The listing builds one solid part. Answer for the finished solid, in the listing's coordinates (mm). Coordinates: 2 decimals unless noted, no trailing zeros. Order: outer loops, then holes, each group sorted by start corner. A loop starts at its lowest first (then second) coordinate and runs counter-clockwise, first axis right, second up. Notation, with made-up numbers: (77.25, 14) -> (93.25, 14) arc R14 cw to (93.25, 28) -> close; hole circle Ø5 at (47.5, 33). An arc over 180 degrees is marked (long way). One line per question, with ' | ' between items.
from build123d import *

# Parameters (mm, degrees)
BOSS_EXTRUDE1_DEPTH    = 25.4
CUT_EXTRUDE1_DEPTH     = 25.4
F_1_1_DIAMETER_HOLE1_D = 25.4


with BuildPart() as part:
    # Sketch1 → Boss-Extrude1 (new body)
    with BuildSketch(Plane.XY):
        with BuildLine():
            Line((-196.85, -171.45), (196.85, -171.45))
            ThreePointArc((196.85, -171.45), (220.423172318, -161.685672318), (230.1875, -138.1125))
            Line((230.1875, -138.1125), (230.1875, 138.1125))
            ThreePointArc((230.1875, 138.1125), (220.423172318, 161.685672318), (196.85, 171.45))
            Line((196.85, 171.45), (-196.85, 171.45))
            ThreePointArc((-196.85, 171.45), (-220.423172318, 161.685672318), (-230.1875, 138.1125))
            Line((-230.1875, 138.1125), (-230.1875, -138.1125))
            ThreePointArc((-230.1875, -138.1125), (-220.423172318, -161.685672318), (-196.85, -171.45))
        make_face()
    extrude(amount=BOSS_EXTRUDE1_DEPTH)

    # Sketch2 → Cut-Extrude1 (cut)
    with BuildSketch(Plane.XY.offset(25.4)):
        with BuildLine():
            Line((-230.1875, 138.1125), (-230.1875, -138.1125))
            ThreePointArc((-230.1875, -138.1125), (-220.423172318, -161.685672318), (-196.85, -171.45))
            Line((-196.85, -171.45), (-122.025168103, -171.45))
            ThreePointArc((-122.025168103, -171.45), (-145.59834042, -161.685672318), (-155.362668103, -138.1125))
            Line((-155.362668103, -138.1125), (-155.362668103, 139.975839194))
            ThreePointArc((-155.362668103, 139.975839194), (-145.020467472, 162.332230308), (-122.137381725, 171.45))
            Line((-122.137381725, 171.45), (-155.460095347, 171.45))
            Line((-155.460095347, 171.45), (-196.85, 171.45))
            ThreePointArc((-196.85, 171.45), (-220.423172318, 161.685672318), (-230.1875, 138.1125))
        make_face()
    extrude(amount=-CUT_EXTRUDE1_DEPTH, mode=Mode.SUBTRACT)

    # 1 (1) Diameter Hole1 (through all)
    with Locations(Plane.XY.offset(25.4)):
        with Locations((25.4, 0), (-36.924961559, 107.95), (87.724961559, 107.95), (150.049923118, 0), (87.724961559, -107.95), (-36.924961559, -107.95), (-99.249923118, 0)):
            Hole(F_1_1_DIAMETER_HOLE1_D / 2)


solid = part.part
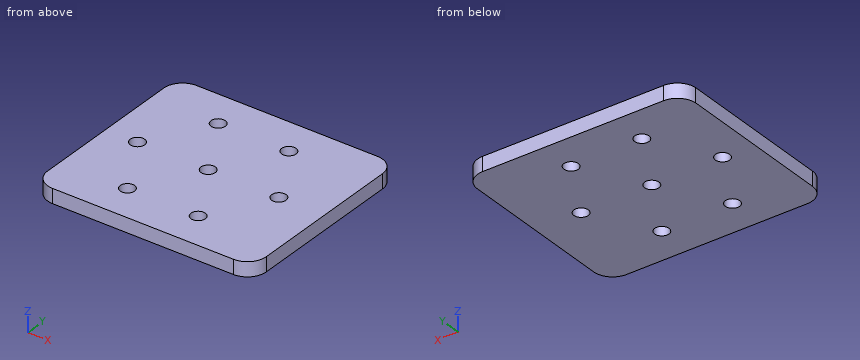
Item 1: Section A-A, the plane x = 25.4 is taken. Give the vertices of the cut face in (y, z).
Computed values:
outline: (-171.45, 0) -> (-12.7, 0) -> (-12.7, 25.4) -> (-171.45, 25.4) -> close; (12.7, 0) -> (171.45, 0) -> (171.45, 25.4) -> (12.7, 25.4) -> close
Item 2: This flat-tipped pin is pushed along its axis until it touches: pin 1 Ø20.5 at (x, y) = (-36.92, 107.95) entering from +Z. Where does it stop, or does it pass through?
Computed values:
pin 1: passes through
Item 3: Section B-B, the plane y = -107.95 is taken. Give the vertices of the cut face in (x, z), plus the area to 3 significant figures.
Computed values:
outline: (-155.36, 0) -> (-49.62, 0) -> (-49.62, 25.4) -> (-155.36, 25.4) -> close; (-24.22, 0) -> (75.02, 0) -> (75.02, 25.4) -> (-24.22, 25.4) -> close; (100.42, 0) -> (230.19, 0) -> (230.19, 25.4) -> (100.42, 25.4) -> close | area: 8,500 mm^2
Item 4: Section C-C, the plane z = 15 is taken. Count the separate pieces of the cut face and the enclosed holes in it, plus the area to 3 significant figures.
Computed values:
separate pieces: 1 | enclosed holes: 7 | area: 128,000 mm^2
Item 5: Section D-D, the plane y = 100 is taken. Give the vertices of the cut face in (x, z).
Computed values:
outline: (-155.36, 0) -> (-46.83, 0) -> (-46.83, 25.4) -> (-155.36, 25.4) -> close; (-27.02, 0) -> (77.82, 0) -> (77.82, 25.4) -> (-27.02, 25.4) -> close; (97.63, 0) -> (230.19, 0) -> (230.19, 25.4) -> (97.63, 25.4) -> close
Item 6: Find the intervals of material crossed by L1, parallel to Y at x = 151, z = 10.5; L2, parallel to X at y = 116.5, z = 2.5; L3, parallel to X at y = 7, z = 5.5, in increasing order.
Computed values:
L1: y = -171.45 to -12.66, 12.66 to 171.45 | L2: x = -155.36 to -46.32, -27.53 to 78.33, 97.12 to 230.19 | L3: x = -155.36 to -109.85, -88.65 to 14.8, 36 to 139.45, 160.65 to 230.19
